```python
from build123d import *

# Parameters (mm, degrees)
ESBO_O1_W                = 38.4
ESBO_O1_H                = 8.4
RESSALTO_EXTRUS_O1_DEPTH = 2.4
ESBO_O2_W                = 1.6
ESBO_O2_H                = 1.6
CORTE_EXTRUS_O1_DEPTH    = 2.5
PADR_O_LINEAR1_COUNT     = 16
PADR_O_LINEAR1_PITCH     = 2.56
ESBO_O3_R                = 0.51
CORTE_EXTRUS_O2_DEPTH    = 21.228939666
PADR_O_LINEAR2_COUNT     = 15
PADR_O_LINEAR2_PITCH     = 2.543
ESBO_O6_W                = 18.080220827
ESBO_O6_H                = 8.4
CORTE_EXTRUS_O3_DEPTH    = 10
ESBO_O8_W                = 12.799779173
ESBO_O8_H                = 8.4
CORTE_EXTRUS_O4_DEPTH    = 10


with BuildPart() as part:
    # Esboço1 → Ressalto-extrusão1 (new body)
    with BuildSketch(Plane.XY):
        Rectangle(ESBO_O1_W, ESBO_O1_H)
    extrude(amount=RESSALTO_EXTRUS_O1_DEPTH)

    # Esboço2 → Corte-extrusão1 (cut)
    with BuildSketch(Plane(origin=(0, 4.2, 0), x_dir=(1, 0, 0), z_dir=(0, 1, 0))):
        with Locations((-18, -1.2)):
            Rectangle(ESBO_O2_W, ESBO_O2_H)
    corte_extrus_o1 = extrude(amount=-CORTE_EXTRUS_O1_DEPTH, mode=Mode.SUBTRACT)

    # Padrão linear1: Corte-extrusão1 ×16
    with Locations(*[(i * PADR_O_LINEAR1_PITCH, 0, 0) for i in range(1, PADR_O_LINEAR1_COUNT)]):
        add(corte_extrus_o1, mode=Mode.SUBTRACT)

    # Esboço3 → Corte-extrusão2 (cut, through all)
    with BuildSketch(Plane(origin=(0, 1.7, 0), x_dir=(1, 0, 0), z_dir=(0, 1, 0))):
        with Locations(Location((-18, -1.2, 0), (0, 0, 270))):
            Circle(ESBO_O3_R)
    corte_extrus_o2 = extrude(amount=-CORTE_EXTRUS_O2_DEPTH, mode=Mode.SUBTRACT)

    # Padrão linear2: Corte-extrusão2 ×15
    with Locations(*[(i * PADR_O_LINEAR2_PITCH, 0, 0) for i in range(1, PADR_O_LINEAR2_COUNT)]):
        add(corte_extrus_o2, mode=Mode.SUBTRACT)

    # Esboço6 → Corte-extrusão3 (cut)
    with BuildSketch(Plane.XY.offset(2.4)):
        with Locations((10.159889587, 0)):
            Rectangle(ESBO_O6_W, ESBO_O6_H)
    extrude(amount=-CORTE_EXTRUS_O3_DEPTH, mode=Mode.SUBTRACT)

    # Esboço8 → Corte-extrusão4 (cut)
    with BuildSketch(Plane.XY.offset(2.4)):
        with Locations((-5.280110414, 0)):
            Rectangle(ESBO_O8_W, ESBO_O8_H)
    extrude(amount=-CORTE_EXTRUS_O4_DEPTH, mode=Mode.SUBTRACT)


solid = part.part
```
Here's how the part is built. I have some questions about the finished solid (model axes, mm). A direction names the side the tool comes from. Round coordinates to 2 decimals unless told otherwise and drop trailing zeros. Loops run counter-clockwise (first coordinate to the right, second up) from the corner with the lowest first, then second, coordinate; pieces in that order, holes last. Notation, with made-up numbers: (31, -31.5) -> (66, -31.5) arc R12 cw to (66, -18.5) -> close; hole circle Ø2 at (89.25, -6.75). An arc over 180 degrees is marked (long way). Answer as CSV lines item,"result". Start each with the question number.
1. I'm going to push flat-ended pins straight in: P1, Ø1.2, axis at x = -18, z = 1.2, coming from the +Y side; P2, Ø1.3, axis at x = -17.5, y = 3, coming from the -Z side. Where does each tip first touch, or does it pass through?
2. Imagine slicing it at D-D on x = -12.75. Write out the boundary of the cut face in (y, z), plus the area to 3 significant figures.
3. If we mould it in two halves opening along Z, with no side actions, what happens to faces 1 (the face through (-15, -4.2, 2)), 2 (the face through (-18, 3, 0.4)), 3 (the face through (-15, 0, 2.4))? For each: pulls with the +Z half, pulls with the -Z half, needs draft (parallel to the pull), parting line crosses it, or undercut.
4. Imagine slicing it at C-C on y = 2.25. Write out the boundary of the cut face in (x, z), plus the area to 3 significant figures.
5. For faces 4 (the face through (-19.2, 0, 1)), 5 (the face through (-18.8, 3, 1)), which set-ups out of +Z, -Z, +X, -X, +Y, -Y let a thin tool reach every point of the face, with its end or its side?
6. I need wall thicknesses on probe 1 along X at (y, z) = (-1.55, 1.2); probe 2 along X at (y, z) = (1.75, 1.35); probe 3 along Z at (x, y) = (-15.5, 0). Which ranges of each line are inside material? Lowest first, please. Write a range as from..to.
7. Imagine slicing it at A-A on z = 1.2. Write out the boundary of the cut face in (x, y), plus the area to 3 significant figures.
8. Imagine slicing it at B-B on x = -18. Write out the boundary of the cut face in (y, z).
Solution:
1,P1,"y = 1.7"
1,P2,"z = 0"
2,outline,"(-4.2, 0) -> (4.2, 0) -> (4.2, 0.4) -> (1.7, 0.4) -> (1.7, 0.72) -> (-4.2, 0.72) -> close; (-4.2, 1.68) -> (1.7, 1.68) -> (1.7, 2) -> (4.2, 2) -> (4.2, 2.4) -> (-4.2, 2.4) -> close"
2,area,"10.5 mm²"
3,face 1,"needs draft"
3,face 2,"undercut"
3,face 3,"pulls with the +Z half"
4,outline,"(-19.2, 0) -> (-11.68, 0) -> (-11.68, 2.4) -> (-19.2, 2.4) -> close; hole (-18.8, 0.4) -> (-17.2, 0.4) -> (-17.2, 2) -> (-18.8, 2) -> close; hole (-16.24, 0.4) -> (-14.64, 0.4) -> (-14.64, 2) -> (-16.24, 2) -> close; hole (-13.68, 0.4) -> (-12.08, 0.4) -> (-12.08, 2) -> (-13.68, 2) -> close"
4,area,"10.4 mm²"
5,face 4,"+Z, -Z, -X, +Y, -Y"
5,face 5,"+Y"
6,probe 1,"-19.2..-18.51, -17.49..-15.97, -14.95..-13.42, -12.4..-11.68"
6,probe 2,"-19.2..-18.8, -17.2..-16.24, -14.64..-13.68, -12.08..-11.68"
6,probe 3,"0..0.69, 1.71..2.4"
7,outline,"(-19.2, -4.2) -> (-18.51, -4.2) -> (-18.51, 1.7) -> (-18.8, 1.7) -> (-18.8, 4.2) -> (-19.2, 4.2) -> close; (-17.49, -4.2) -> (-15.97, -4.2) -> (-15.97, 1.7) -> (-16.24, 1.7) -> (-16.24, 4.2) -> (-17.2, 4.2) -> (-17.2, 1.7) -> (-17.49, 1.7) -> close; (-14.95, -4.2) -> (-13.42, -4.2) -> (-13.42, 1.7) -> (-13.68, 1.7) -> (-13.68, 4.2) -> (-14.64, 4.2) -> (-14.64, 1.7) -> (-14.95, 1.7) -> close; (-12.4, -4.2) -> (-11.68, -4.2) -> (-11.68, 4.2) -> (-12.08, 4.2) -> (-12.08, 1.7) -> (-12.4, 1.7) -> close"
7,area,"33.1 mm²"
8,outline,"(-4.2, 0) -> (4.2, 0) -> (4.2, 0.4) -> (1.7, 0.4) -> (1.7, 0.69) -> (-4.2, 0.69) -> close; (-4.2, 1.71) -> (1.7, 1.71) -> (1.7, 2) -> (4.2, 2) -> (4.2, 2.4) -> (-4.2, 2.4) -> close"
